Can you work these out from the drawing? Everything is in mm from the part's minimum corner. Round coordinates to 2 decimals unless told otherwise and drop trailing zeros. Order: outer loops, then holes, each group sorted by start corner. A loop starts at its lowest first (then second) coordinate and runs counter-clockwise, first axis right, second up. Notation, with made-up numbers: (38.5, -29) - (85.5, -29) arc R15 cw to (85.5, -25) - close; hole circle Ø8 at (17.25, 63.25). An arc over 180 degrees is marked (long way). Write item = value, one per line.
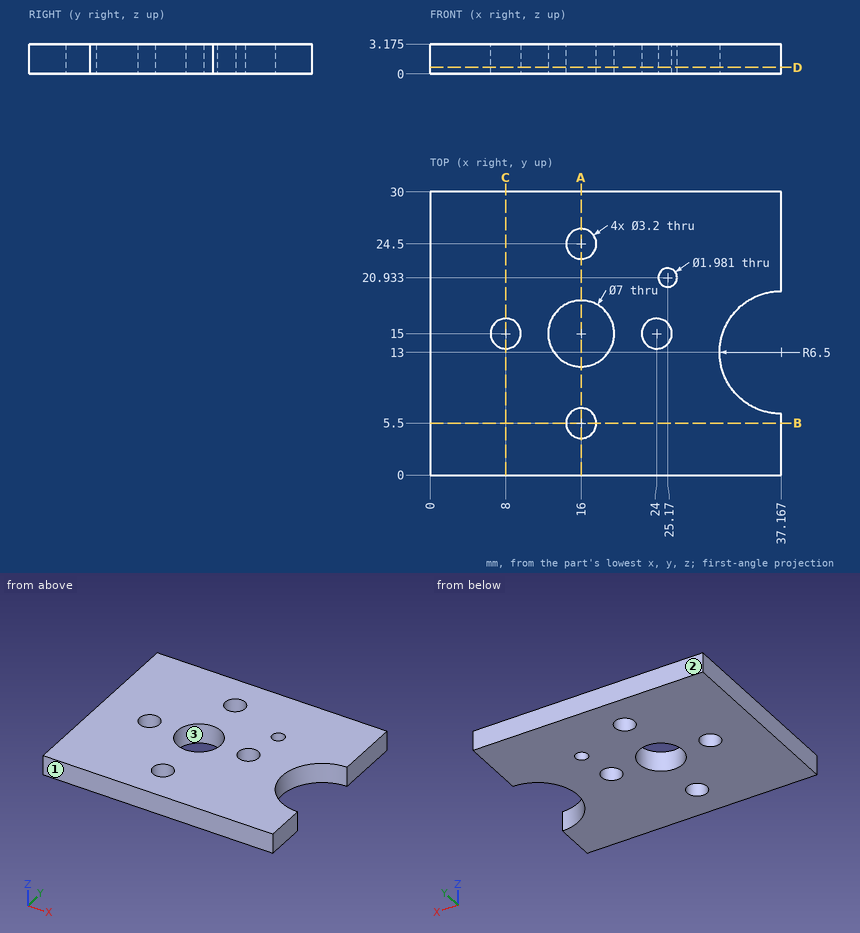
(1) Will these pins go through, and if not, where does the flat tip stop? P1, Ø12, axis at x = 28, y = 23, coming from the -Z side; P2, Ø6.5, axis at x = 16, y = 15, coming from the +Z side.
Computed:
P1 = 0
P2 = through
(2) If we section it at D-D (z = 0.7): Write out the boundary of the cut face in (x, y).
Computed:
outline = (0, 0) - (37.17, 0) - (37.17, 6.5) arc R6.5 cw to (37.17, 19.5) - (37.17, 30) - (0, 30) - close; hole circle Ø3.2 at (8, 15); hole circle Ø7 at (16, 15); hole circle Ø3.2 at (16, 5.5); hole circle Ø3.2 at (16, 24.5); hole circle Ø3.2 at (24, 15); hole circle Ø1.98 at (25.17, 20.93)
(3) If we section it at A-A (x = 16): Write out the boundary of the cut face in (y, z) (1 decimal).
Computed:
outline = (0, 0) - (3.9, 0) - (3.9, 3.2) - (0, 3.2) - close; (7.1, 0) - (11.5, 0) - (11.5, 3.2) - (7.1, 3.2) - close; (18.5, 0) - (22.9, 0) - (22.9, 3.2) - (18.5, 3.2) - close; (26.1, 0) - (30, 0) - (30, 3.2) - (26.1, 3.2) - close
(4) Thinking about a two-plate mould opening in Y: for the marked faces 1, 2 and 3, which applies, +Y half, -Y half, draft (parallel to the pull), parting line (faces both ways), or undercut?
Computed:
face_1 = -Y half
face_2 = +Y half
face_3 = undercut
(5) If I drill on line 1 (X direction, y = 5.5, z = 2.15); line 2 (Y direction, x = 16, z = 1.55); line 3 (Y direction, x = 8, z = 1), over which ranges is the centre line in solid material (lowest first)? Write a range as from..to.
Computed:
line_1 = 0..14.4, 17.6..37.17
line_2 = 0..3.9, 7.1..11.5, 18.5..22.9, 26.1..30
line_3 = 0..13.4, 16.6..30
(6) If we section it at B-B (y = 5.5): Write out the boundary of the cut face in (x, z) (1 decimal).
Computed:
outline = (0, 0) - (14.4, 0) - (14.4, 3.2) - (0, 3.2) - close; (17.6, 0) - (37.2, 0) - (37.2, 3.2) - (17.6, 3.2) - close
(7) If we section it at C-C (x = 8): Write out the boundary of the cut face in (y, z) (1 decimal).
Computed:
outline = (0, 0) - (13.4, 0) - (13.4, 3.2) - (0, 3.2) - close; (16.6, 0) - (30, 0) - (30, 3.2) - (16.6, 3.2) - close
